from build123d import *

# Parameters (mm, degrees)
SKETCH1_W           = 120
SKETCH1_H           = 134.5
BOSS_EXTRUDE1_DEPTH = 3.175
CUT_EXTRUDE1_REACH  = 92.181
SKETCH2_W           = 11.91979388
SKETCH2_H           = 134.5
SKETCH2_R           = 2.75


with BuildPart() as part:
    # Sketch1 → Boss-Extrude1 (new body)
    with BuildSketch(Plane.XY):
        Rectangle(SKETCH1_W, SKETCH1_H)
    extrude(amount=BOSS_EXTRUDE1_DEPTH)

    # Sketch2 → Cut-Extrude1 (cut, up to next)
    with BuildSketch(Plane.XY.offset(3.175), mode=Mode.PRIVATE) as cut_extrude1_sk1:
        with Locations((-54.04010306, 0)):
            Rectangle(SKETCH2_W, SKETCH2_H)
    cut_extrude1_tool1 = extrude(cut_extrude1_sk1.sketch, amount=-CUT_EXTRUDE1_REACH, mode=Mode.PRIVATE) & part.part
    # Sketch2 → Cut-Extrude1 (cut, up to next)
    with BuildSketch(Plane.XY.offset(3.175), mode=Mode.PRIVATE) as cut_extrude1_sk2:
        with Locations((-44.08020612, 62.25)):
            Circle(SKETCH2_R)
    cut_extrude1_tool2 = extrude(cut_extrude1_sk2.sketch, amount=-CUT_EXTRUDE1_REACH, mode=Mode.PRIVATE) & part.part
    # Sketch2 → Cut-Extrude1 (cut, up to next)
    with BuildSketch(Plane.XY.offset(3.175), mode=Mode.PRIVATE) as cut_extrude1_sk3:
        with Locations((56, -62.25)):
            Circle(SKETCH2_R)
    cut_extrude1_tool3 = extrude(cut_extrude1_sk3.sketch, amount=-CUT_EXTRUDE1_REACH, mode=Mode.PRIVATE) & part.part
    # Sketch2 → Cut-Extrude1 (cut, up to next)
    with BuildSketch(Plane.XY.offset(3.175), mode=Mode.PRIVATE) as cut_extrude1_sk4:
        with Locations((-44.08020612, -62.25)):
            Circle(SKETCH2_R)
    cut_extrude1_tool4 = extrude(cut_extrude1_sk4.sketch, amount=-CUT_EXTRUDE1_REACH, mode=Mode.PRIVATE) & part.part
    # Sketch2 → Cut-Extrude1 (cut, up to next)
    with BuildSketch(Plane.XY.offset(3.175), mode=Mode.PRIVATE) as cut_extrude1_sk5:
        with Locations((56, 62.25)):
            Circle(SKETCH2_R)
    cut_extrude1_tool5 = extrude(cut_extrude1_sk5.sketch, amount=-CUT_EXTRUDE1_REACH, mode=Mode.PRIVATE) & part.part
    add(cut_extrude1_tool1.solids().sort_by_distance((-54.040103, 0, 3.175))[0], mode=Mode.SUBTRACT)
    add(cut_extrude1_tool2.solids().sort_by_distance((-44.080206, 62.25, 3.175))[0], mode=Mode.SUBTRACT)
    add(cut_extrude1_tool3.solids().sort_by_distance((56, -62.25, 3.175))[0], mode=Mode.SUBTRACT)
    add(cut_extrude1_tool4.solids().sort_by_distance((-44.080206, -62.25, 3.175))[0], mode=Mode.SUBTRACT)
    add(cut_extrude1_tool5.solids().sort_by_distance((56, 62.25, 3.175))[0], mode=Mode.SUBTRACT)


solid = part.part
Check sheet for the modelled part. Datum: model origin and axes. Units: mm. Give positions to 0.01 mm unless a question says otherwise; leave off trailing zeros. Write each loop counter-clockwise with the first axis right and the second up, starting at its lowest first coordinate (ties: lowest second). Pieces come first, ordered by that corner, then holes. Notation, with made-up numbers: (43, 86.5) -> (54, 86.5) arc R24 cw to (54, 118.5) -> close; hole circle Ø4 at (4.25, -4.5). An arc over 180 degrees is marked (long way). Write item = value, one per line.
Item 1: Sectioned sample at A-A on x = 56. Record the boundary of the cut face in (y, z) (3 decimals), and give its area (3 significant figures).
Output:
outline = (-67.25, 0) -> (-65, 0) -> (-65, 3.175) -> (-67.25, 3.175) -> close; (-59.5, 0) -> (59.5, 0) -> (59.5, 3.175) -> (-59.5, 3.175) -> close; (65, 0) -> (67.25, 0) -> (67.25, 3.175) -> (65, 3.175) -> close
area = 392 mm^2
Item 2: Release check for a two-part mould opening along X. For faces 1 (the flat face through (5, -67.25, 2)), 2 (the cylindrical face through (53.973, 64.109, 1.61)), 3 (the flat face through (60, -1, 2)) record: +X half, -X half, draft (parallel to the pull), parting line (faces both ways), or undercut.
Output:
face_1 = draft
face_2 = undercut
face_3 = +X half
Item 3: Sectioned sample at B-B on y = -62.25. Record the boundary of the cut face in (x, z) (3 decimals), and give its area (3 significant figures).
Output:
outline = (-48.08, 0) -> (-46.83, 0) -> (-46.83, 3.175) -> (-48.08, 3.175) -> close; (-41.33, 0) -> (53.25, 0) -> (53.25, 3.175) -> (-41.33, 3.175) -> close; (58.75, 0) -> (60, 0) -> (60, 3.175) -> (58.75, 3.175) -> close
area = 308 mm^2
Item 4: Scan line: probe 1 along Y at (x, z) = (56, 2.2). Record every from-to range of solid material in increasing order. Write a range as from..to.
Output:
probe_1 = -67.25..-65, -59.5..59.5, 65..67.25
Item 5: Gauge pin test, flat ends, axial feed: pin 1 (3 mm diameter, centred on x = -9.5, y = 42.5, fed in from -Z); pin 2 (5 mm diameter, centred on x = 56, y = 62.25, fed in from +Z). Record the tip position at first contact, or that the pin passes through.
Output:
pin_1 = 0
pin_2 = through
